Design review of the part shown in the three views and the two pictorial views. Dimensions are in mm from the part's minimum x, y and z. A direction names the side the tool comes from. Coordinates: 2 decimals unless noted, no trailing zeros. Write each loop counter-clockwise with the first axis right and the second up, starting at its lowest first coordinate (ties: lowest second). Pieces come first, ordered by that corner, then holes. Notation, with made-up numbers: (-36, 54) -> (-4, 54) arc R16 ccw to (-4, 72) -> close; hole circle Ø2 at (33, -15). An arc over 180 degrees is marked (long way). Answer in a Markdown table with one row per item. Add a question column.
Item 1: For the marked faces 4, 5 and 6, list the 3-axis set-ups (+Z, -Z, +X, -X, +Y, -Y) from which the entire face can be reached by the end or side of a thin tool; tool diameter is ignored.
Item 2: Take a section at B-B, the plane z = 38.1. Write out the cut boundary in (x, y), and give its area (3 significant figures).
Item 3: Take a section at D-D, the plane x = 160.5. Write out the cut boundary in (y, z), and give its area (3 significant figures).
Item 4: Take a section at C-C, the plane y = 31.75. Write out the cut boundary in (x, z), and give its area (3 significant figures).
Item 5: To check wall thickness, follow line 1 (Y direction, x = 167, z = 38.1); line 2 (X direction, y = 158, z = 62.5); line 3 (Z direction, x = 162, y = 171). State the ranges of each line that lie inside material, in increasing order.
Item 6: Clearance check with flat-ended pins moving along their axes: P1, Ø3, axis at y = 107, z = 63.5, coming from the -X side; P2, Ø10, axis at x = 124.5, z = 53, coming from the -Y side; P3, Ø4, axis at x = 136.5, z = 10.5, coming from the +Y side. State where each tip first meets the part, or that it passes through.
Item 7: Draft analysis for pull direction Z (two halves, no side actions). For the marked faces 1, 2 and 3, state which applies: released by +Z, released by -Z, zero draft, split by the parting line, or undercut.
Item 8: Take a section at A-A, the plane y = 142. Write out the cut boundary in (x, z).
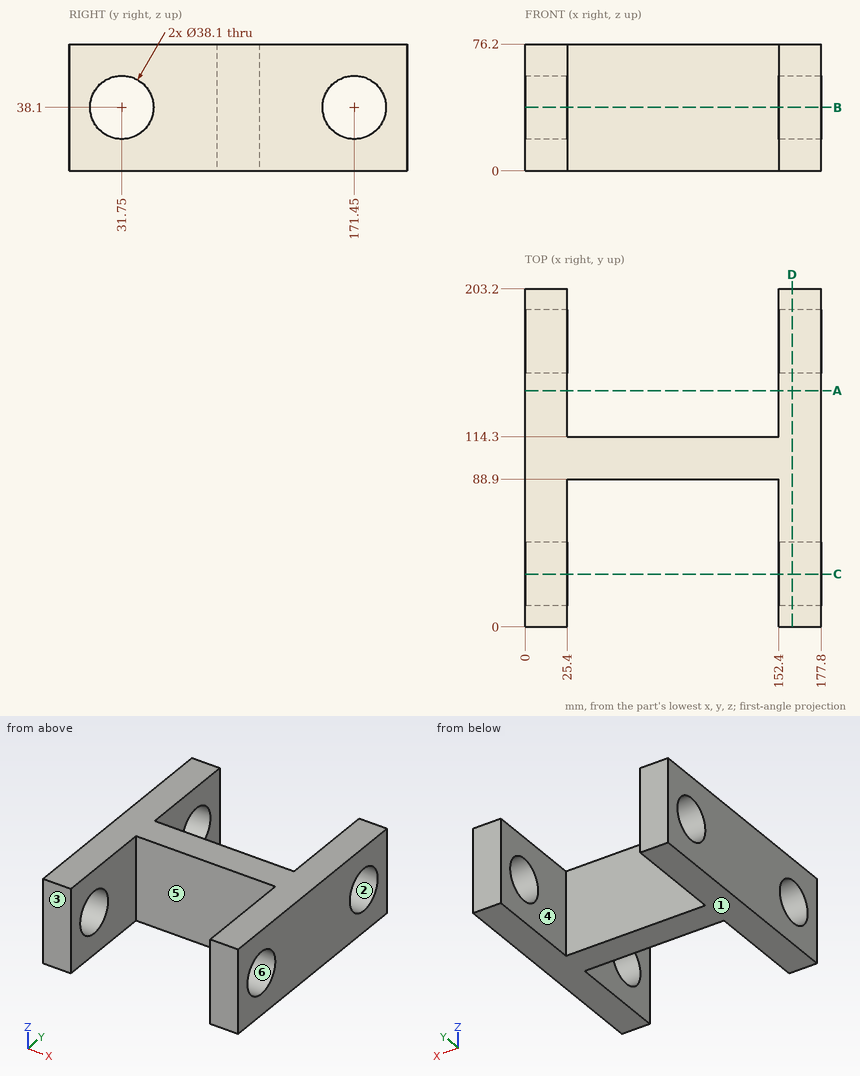
Answers:
| question | item | result |
|---|---|---|
| 1 | face 4 | +Z, -Z, +Y |
| 1 | face 5 | +Z, -Z, -Y |
| 1 | face 6 | +X, -X |
| 2 | outline | (0, 0) -> (25.4, 0) -> (25.4, 12.7) -> (0, 12.7) -> close; (0, 50.8) -> (25.4, 50.8) -> (25.4, 88.9) -> (152.4, 88.9) -> (152.4, 50.8) -> (177.8, 50.8) -> (177.8, 152.4) -> (152.4, 152.4) -> (152.4, 114.3) -> (25.4, 114.3) -> (25.4, 152.4) -> (0, 152.4) -> close; (0, 190.5) -> (25.4, 190.5) -> (25.4, 203.2) -> (0, 203.2) -> close; (152.4, 0) -> (177.8, 0) -> (177.8, 12.7) -> (152.4, 12.7) -> close; (152.4, 190.5) -> (177.8, 190.5) -> (177.8, 203.2) -> (152.4, 203.2) -> close |
| 2 | area | 9,680 mm^2 |
| 3 | outline | (0, 0) -> (203.2, 0) -> (203.2, 76.2) -> (0, 76.2) -> close; hole circle Ø38.1 at (31.75, 38.1); hole circle Ø38.1 at (171.45, 38.1) |
| 3 | area | 13,200 mm^2 |
| 4 | outline | (0, 0) -> (25.4, 0) -> (25.4, 19.05) -> (0, 19.05) -> close; (0, 57.15) -> (25.4, 57.15) -> (25.4, 76.2) -> (0, 76.2) -> close; (152.4, 0) -> (177.8, 0) -> (177.8, 19.05) -> (152.4, 19.05) -> close; (152.4, 57.15) -> (177.8, 57.15) -> (177.8, 76.2) -> (152.4, 76.2) -> close |
| 4 | area | 1,940 mm^2 |
| 5 | line 1 | y = 0 to 12.7, 50.8 to 152.4, 190.5 to 203.2 |
| 5 | line 2 | x = 0 to 25.4, 152.4 to 177.8 |
| 5 | line 3 | z = 0 to 19.06, 57.14 to 76.2 |
| 6 | P1 | stops at x = 0 |
| 6 | P2 | stops at y = 88.9 |
| 6 | P3 | stops at y = 114.3 |
| 7 | face 1 | released by -Z |
| 7 | face 2 | undercut |
| 7 | face 3 | zero draft |
| 8 | outline | (0, 0) -> (25.4, 0) -> (25.4, 76.2) -> (0, 76.2) -> close; (152.4, 0) -> (177.8, 0) -> (177.8, 76.2) -> (152.4, 76.2) -> close |
